Verification items for the finished model (mm, model axes). Face numbers are marked on the shaded views. Give positions to 0.01 mm unless a question says otherwise; leave off trailing zeros. Write each loop counter-clockwise with the first axis right and the second up, starting at its lowest first coordinate (ties: lowest second). Pieces come first, ordered by that corner, then holes. Notation, with made-up numbers: (34, -18) -> (39, -18) arc R17 cw to (39, 5) -> close; hole circle Ø1 at (43, 59.25). An arc over 180 degrees is marked (long way). Write item = value, one per line.
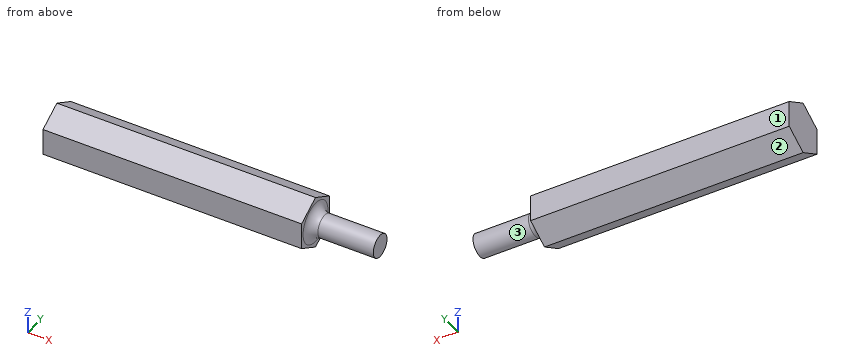
from build123d import *

# Parameters (mm, degrees)
BOSS_EXTRUDE1_DEPTH = 88.9
SKETCH2_R           = 9.399520033
SKETCH2_R_2         = 3.1369
CUT_EXTRUDE1_DEPTH  = 17.78
FILLET1_R           = 2.54


with BuildPart() as part:
    # Sketch1 → Boss-Extrude1 (new body)
    with BuildSketch(Plane(origin=(0, 0, 0), x_dir=(0, 0, -1), z_dir=(1, 0, 0))):
        Polygon((3.666174209, -6.35), (7.332348419, 0), (3.666174209, 6.35), (-3.666174209, 6.35), (-7.332348419, 0), (-3.666174209, -6.35), align=None)
    extrude(amount=BOSS_EXTRUDE1_DEPTH)

    # Sketch2 → Cut-Extrude1 (cut)
    with BuildSketch(Plane(origin=(88.9, 0, 0), x_dir=(0, 0, -1), z_dir=(1, 0, 0))):
        Circle(SKETCH2_R)
        Circle(SKETCH2_R_2, mode=Mode.SUBTRACT)
    extrude(amount=-CUT_EXTRUDE1_DEPTH, mode=Mode.SUBTRACT)

    # Fillet1
    fillet1_edges = [part.edges().sort_by_distance(p)[0] for p in [
        (71.12, 0, 3.1369),
    ]]
    fillet(fillet1_edges, radius=FILLET1_R)


solid = part.part
Item 1: Sectioned sample at B-B on x = 44. Record the cut outline in (y, z).
Response values:
outline = (-6.35, -3.67) -> (0, -7.33) -> (6.35, -3.67) -> (6.35, 3.67) -> (0, 7.33) -> (-6.35, 3.67) -> close
Item 2: Sectioned sample at A-A on z = 0. Record the cut outline in (x, y).
Response values:
outline = (0, -6.35) -> (71.12, -6.35) -> (71.12, -5.68) arc R2.54 cw to (73.66, -3.14) -> (88.9, -3.14) -> (88.9, 3.14) -> (73.66, 3.14) arc R2.54 cw to (71.12, 5.68) -> (71.12, 6.35) -> (0, 6.35) -> close
Item 3: Mould release check, pull along Z, two halves, no side actions. Record for the marked faces 1, 2 and 3: +Z half, -Z half, draft (parallel to the pull), parting line (faces both ways), or undercut.
Response values:
face_1 = draft
face_2 = -Z half
face_3 = parting line
Item 4: Material ranges on line 1 (X direction, y = 6, z = -2.75); line 2 (Z direction, x = 26, y = 1.5); line 3 (Z direction, x = 56, y = -1.75), recorded low to high.
Response values:
line_1 = 0 to 71.12
line_2 = -6.47 to 6.47
line_3 = -6.32 to 6.32
